For this review, take the finished solid that the model builds, in its own axes (mm). Face numbers are marked on the shaded views. A direction names the side the tool comes from. Give positions to 0.01 mm unless a question says otherwise; leave off trailing zeros. Write each loop counter-clockwise with the first axis right and the second up, starting at its lowest first coordinate (ties: lowest second). Pieces come first, ordered by that corner, then holes. Notation, with made-up numbers: M -39,20 L -23,20 A12 ccw -23,35 Z; hole C -14,-17 d10. An arc over 180 degrees is marked long. One line per item, written item: value. Start each with the question number.
Item 1: Consider section B-B, the plane x = 7. Write out the cut boundary in (y, z), and give its area (3 significant figures).
Item 2: Consider section A-A, the plane z = 22. Write out the cut boundary in (x, y).
Item 3: Tool access review of the marked faces 1 and 2: name each direction out of +Z, -Z, +X, -X, +Y, -Y from which nothing blocks a thin tool from reaching the whole face with its end or side.
Item 4: Consider section C-C, the plane y = 2. Write out the cut boundary in (x, z).
Item 5: To check wall thickness, follow probe 1 along Y at (x, z) = (-24, 14); probe 2 along Y at (x, z) = (-19.5, 64). State the ranges of each line that lie inside material, in increasing order.
Item 6: Mouldability with a two-part tool opening along Z and no side actions: class the marked faces 3, 4 and 5 as released by +Z, released by -Z, zero draft, split by the parting line, or undercut.
Item 7: Clearance check with flat-ended pins moving along their axes: pin 1 Ø0.6 at (x, z) = (-40.5, 49.5) entering from +Y; pin 2 Ø8 at (x, y) = (-0.5, 19.5) entering from +Z. State where each tip first meets the part, or that it passes through.
```python
from build123d import *

# Parameters (mm, degrees)
SKETCH1_W           = 85
SKETCH1_H           = 85
BOSS_EXTRUDE1_DEPTH = 85
FILLET1_R           = 10
SHELL1_T            = 2
CUT_EXTRUDE1_REACH  = 106.103
BOSS_EXTRUDE2_DEPTH = 20
SKETCH4_W           = 2
SKETCH4_H           = 10
BOSS_EXTRUDE3_DEPTH = 0.5
CIRPATTERN1_COUNT   = 4


with BuildPart() as part:
    # Sketch1 → Boss-Extrude1 (new body)
    with BuildSketch(Plane.XY):
        Rectangle(SKETCH1_W, SKETCH1_H)
    extrude(amount=BOSS_EXTRUDE1_DEPTH)

    # Fillet1
    fillet1_edges = [part.edges().sort_by_distance(p)[0] for p in [
        (42.5, -42.5, 42.5),
        (-42.5, -42.5, 42.5),
        (-42.5, 42.5, 42.5),
        (42.5, 42.5, 42.5),
    ]]
    fillet(fillet1_edges, radius=FILLET1_R)

    # Shell1 (no face opened: a closed hollow body)
    add(offset(amount=-SHELL1_T, mode=Mode.PRIVATE), mode=Mode.SUBTRACT)

    # Sketch2 → Cut-Extrude1 (cut, up to next)
    with BuildSketch(Plane.XY.offset(85), mode=Mode.PRIVATE) as cut_extrude1_sk1:
        with BuildLine():
            Line((32.5, 35.5), (-32.5, 35.5))
            ThreePointArc((-32.5, 35.5), (-34.621320344, 34.621320344), (-35.5, 32.5))
            Line((-35.5, 32.5), (-35.5, -32.5))
            ThreePointArc((-35.5, -32.5), (-34.621320344, -34.621320344), (-32.5, -35.5))
            Line((-32.5, -35.5), (32.5, -35.5))
            ThreePointArc((32.5, -35.5), (34.621320344, -34.621320344), (35.5, -32.5))
            Line((35.5, -32.5), (35.5, 32.5))
            ThreePointArc((35.5, 32.5), (34.621320344, 34.621320344), (32.5, 35.5))
        make_face()
    cut_extrude1_tool1 = extrude(cut_extrude1_sk1.sketch, amount=-CUT_EXTRUDE1_REACH, mode=Mode.PRIVATE) & part.part
    add(cut_extrude1_tool1.solids().sort_by_distance((0, 0, 85))[0], mode=Mode.SUBTRACT)

    # Sketch3 → Boss-Extrude2 (add)
    with BuildSketch(Plane(origin=(0, 0, 83), x_dir=(-1, 0, 0), z_dir=(0, 0, -1))):
        with BuildLine():
            Line((-32.5, 40.5), (32.5, 40.5))
            ThreePointArc((32.5, 40.5), (38.156854249, 38.156854249), (40.5, 32.5))
            Line((40.5, 32.5), (40.5, -32.5))
            ThreePointArc((40.5, -32.5), (38.156854249, -38.156854249), (32.5, -40.5))
            Line((32.5, -40.5), (-32.5, -40.5))
            ThreePointArc((-32.5, -40.5), (-38.156854249, -38.156854249), (-40.5, -32.5))
            Line((-40.5, -32.5), (-40.5, 32.5))
            ThreePointArc((-40.5, 32.5), (-38.156854249, 38.156854249), (-32.5, 40.5))
        make_face()
        with BuildLine():
            Line((38.5, -32.5), (38.5, 32.5))
            ThreePointArc((38.5, 32.5), (36.742640687, 36.742640687), (32.5, 38.5))
            Line((32.5, 38.5), (-32.5, 38.5))
            ThreePointArc((-32.5, 38.5), (-36.742640687, 36.742640687), (-38.5, 32.5))
            Line((-38.5, 32.5), (-38.5, -32.5))
            ThreePointArc((-38.5, -32.5), (-36.742640687, -36.742640687), (-32.5, -38.5))
            Line((-32.5, -38.5), (32.5, -38.5))
            ThreePointArc((32.5, -38.5), (36.742640687, -36.742640687), (38.5, -32.5))
        make_face(mode=Mode.SUBTRACT)
    extrude(amount=BOSS_EXTRUDE2_DEPTH)

    # Sketch4 → Boss-Extrude3 (add)
    with BuildSketch(Plane.ZY.offset(-40.5)):
        with Locations((50, 0)):
            Rectangle(SKETCH4_W, SKETCH4_H)
    boss_extrude3 = extrude(amount=BOSS_EXTRUDE3_DEPTH)

    # CirPattern1: Boss-Extrude3 ×4 about axis
    cirpattern1_axis = Axis((0, 0, 0), (0, 0, 1))
    for i in range(1, CIRPATTERN1_COUNT):
        add(boss_extrude3.rotate(cirpattern1_axis, i * 360 / CIRPATTERN1_COUNT))


solid = part.part
```
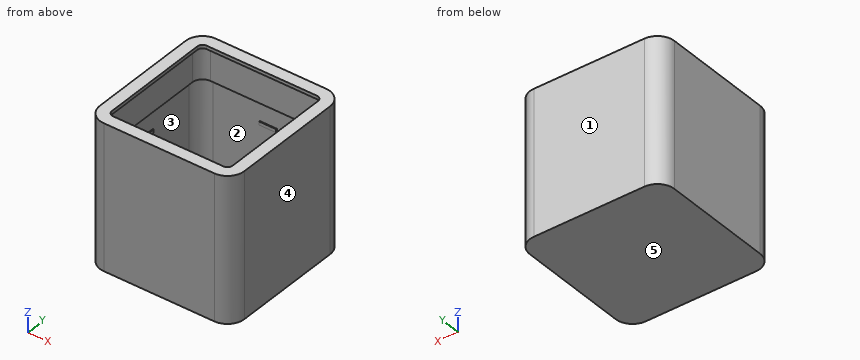
Model answer:
1. outline: M -42.5,0 L 42.5,0 L 42.5,85 L 35.5,85 L 35.5,83 L 38.5,83 L 38.5,63 L 40.5,63 L 40.5,2 L -40.5,2 L -40.5,63 L -38.5,63 L -38.5,83 L -35.5,83 L -35.5,85 L -42.5,85 Z
1. area: 602 mm2
2. outline: M -42.5,-32.5 A10 ccw -32.5,-42.5 L 32.5,-42.5 A10 ccw 42.5,-32.5 L 42.5,32.5 A10 ccw 32.5,42.5 L -32.5,42.5 A10 ccw -42.5,32.5 Z; hole M -40.5,-32.5 A8 ccw -32.5,-40.5 L 32.5,-40.5 A8 ccw 40.5,-32.5 L 40.5,32.5 A8 ccw 32.5,40.5 L -32.5,40.5 A8 ccw -40.5,32.5 Z
3. face 1: +Z, -Z, +X, -X, +Y
3. face 2: none
4. outline: M -42.5,0 L 42.5,0 L 42.5,85 L 35.5,85 L 35.5,83 L 38.5,83 L 38.5,63 L 40.5,63 L 40.5,51 L 40,51 L 40,49 L 40.5,49 L 40.5,2 L -40.5,2 L -40.5,49 L -40,49 L -40,51 L -40.5,51 L -40.5,63 L -38.5,63 L -38.5,83 L -35.5,83 L -35.5,85 L -42.5,85 Z
5. probe 1: y = -42.5 to -40.5, 40.5 to 42.5
5. probe 2: y = -42.5 to -38.5, 38.5 to 42.5
6. face 3: undercut
6. face 4: zero draft
6. face 5: released by -Z
7. pin 1: stops at y = 38.88
7. pin 2: stops at z = 2
